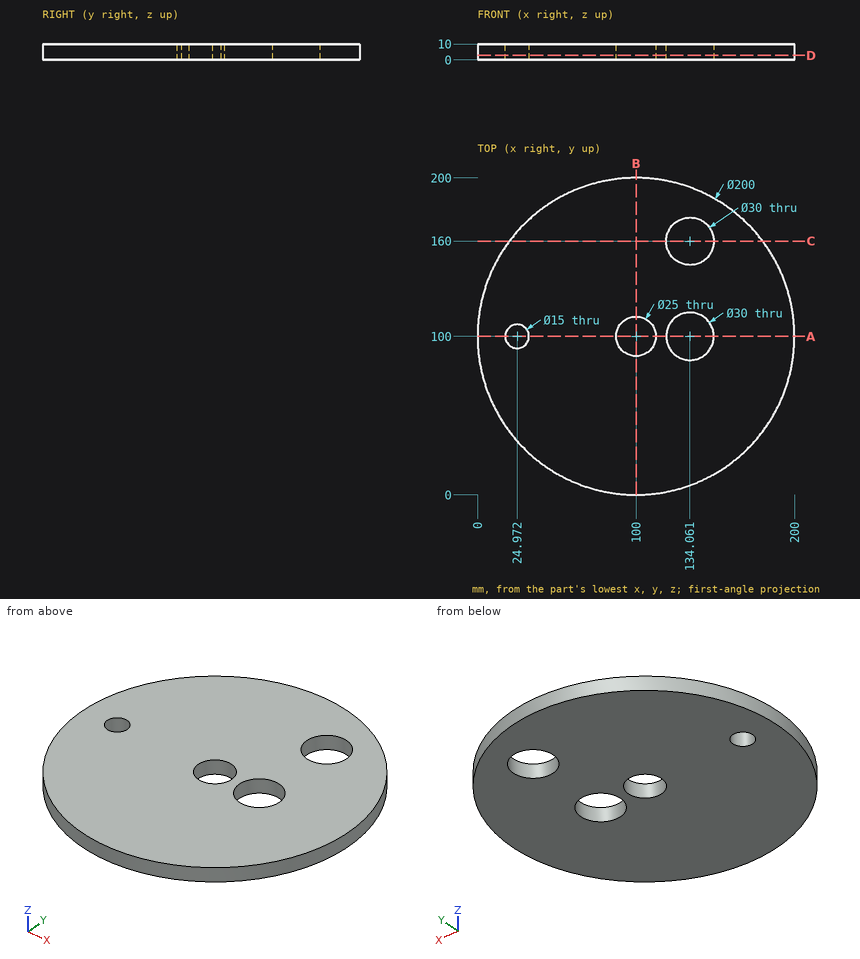
Could you check a few things on this drawing? It's one solid part, dimensions in mm from its lowest x, y, z. Round coordinates to 2 decimals unless told otherwise and drop trailing zeros. Order: outer loops, then holes, each group sorted by start corner. A loop starts at its lowest first (then second) coordinate and runs counter-clockwise, first axis right, second up. Notation, with made-up numbers: M -30.75,28 L -6.75,28 A17 cw -6.75,48 Z; hole C -37.75,77.5 d2. An arc over 180 degrees is marked long. Return JSON: item names as keys, results as strings. Group by question number.
1. If we section it at D-D on z = 2.75: List the corners of the cut face in (x, y) for me.
2. If we section it at C-C on y = 160: List the corners of the cut face in (x, z) for me.
3. Please list where these lines run through material, in increasing order: probe 1 along Y at (x, z) = (134, 9.5); probe 2 along Y at (x, z) = (100, 8.25); probe 3 along Y at (x, z) = (145, 9) (1 decimal).
4. If we section it at B-B on x = 100: List the corners of the cut face in (y, z) for me.
5. I'm going to push flat-ended pins straight in: pin 1 Ø3 at (y, z) = (129.5, 2) entering from +X; pin 2 Ø3 at (x, z) = (90.5, 2.5) entering from +Y; pin 3 Ø24 at (x, y) = (134.06, 100) entering from -Z; pin 4 Ø6 at (x, z) = (178.5, 7) entering from +Y. Where does each tip first touch, or does it pass through?
6. If we section it at A-A on y = 100: List the corners of the cut face in (x, z) for me.
Reply:
{
 "1": {"outline": "C 100,100 d200; hole C 24.97,100 d15; hole C 100,100 d25; hole C 134.06,100 d30; hole C 134.06,160 d30"},
 "2": {"outline": "M 20,0 L 119.06,0 L 119.06,10 L 20,10 Z; M 149.06,0 L 180,0 L 180,10 L 149.06,10 Z"},
 "3": {"probe 1": "5.96 to 85, 115 to 145, 175 to 194.04", "probe 2": "0 to 87.5, 112.5 to 200", "probe 3": "10.7 to 89.7, 110.3 to 149.7, 170.3 to 189.3"},
 "4": {"outline": "M 0,0 L 87.5,0 L 87.5,10 L 0,10 Z; M 112.5,0 L 200,0 L 200,10 L 112.5,10 Z"},
 "5": {"pin 1": "x = 196", "pin 2": "y = 199.68", "pin 3": "through", "pin 4": "y = 165.57"},
 "6": {"outline": "M 0,0 L 17.47,0 L 17.47,10 L 0,10 Z; M 32.47,0 L 87.5,0 L 87.5,10 L 32.47,10 Z; M 112.5,0 L 119.06,0 L 119.06,10 L 112.5,10 Z; M 149.06,0 L 200,0 L 200,10 L 149.06,10 Z"}
}
